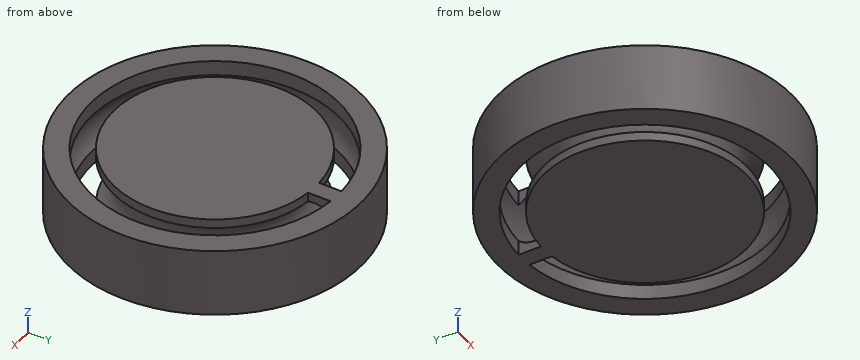
from build123d import *

# Parameters (mm, degrees)
SKETCH_R     = 26
PAD_DEPTH    = 12
POCKET_DEPTH = 12
SKETCH002_R  = 4.5


with BuildPart() as part:
    # Sketch → Pad (new body)
    with BuildSketch(Plane.XY):
        Circle(SKETCH_R)
    extrude(amount=PAD_DEPTH)

    # Sketch001 → Pocket (cut)
    with BuildSketch(Plane.XY):
        with BuildLine():
            ThreePointArc((-1.065198, 21.974197), (-0.435817, -21.995683), (1.934802, 21.914756))
            Line((1.934802, 21.914756), (1.934802, 17.895713))
            ThreePointArc((-1.065198, 17.968454), (-0.436321, -17.994711), (1.934802, 17.895713))
            Line((-1.065198, 21.974197), (-1.065198, 17.968454))
        make_face()
    extrude(amount=POCKET_DEPTH, mode=Mode.SUBTRACT)

    # Sketch002 → Groove (revolve, cut)
    with BuildSketch(Plane.YZ):
        with Locations((19, 6)):
            Circle(SKETCH002_R)
    revolve(axis=Axis((0, 0, 0), (0, 0, 1)), mode=Mode.SUBTRACT)


solid = part.part
Source: CAD feature listing. Evaluate the final solid. Frame: model axes, mm. Give positions to 0.01 mm unless a question says otherwise; leave off trailing zeros. Order: outer loops, then holes, each group sorted by start corner. A loop starts at its lowest first (then second) coordinate and runs counter-clockwise, first axis right, second up. Notation, with made-up numbers: (50.25, 87.25) -> (92.25, 87.25) arc R14 cw to (92.25, 99.25) -> close; hole circle Ø10 at (12.25, 47.5). An arc over 180 degrees is marked (long way). Use a Markdown table: item, result.
1) Section query A-A, the plane z = 3.5. Return the cut outline in (x, y), then the cut area to 3 significant figures.
Answer list:
| item | result |
|---|---|
| outline | circle Ø52 at (0, 0); circle Ø30.52 at (0, 0); hole circle Ø45.48 at (0, 0) |
| area | 1,230 mm² |
2) Contact query for flat-ended pins moving along their axis: P1, Ø3, axis at y = -19, z = 8.5, coming from the -X side; P2, Ø2, axis at x = 13, z = 6, coming from the -Y side; P3, Ø6, axis at x = 1, y = 13, coming from the -Z side; P4, Ø1.3, axis at y = 19, z = 10.5, coming from the +X side. Output: stop coordinate, or through.
Answer list:
| item | result |
|---|---|
| P1 | x = -19.23 |
| P2 | y = -23.07 |
| P3 | z = 0 |
| P4 | x = 18.42 |
3) Section query D-D, the plane z = 7.25. Return the cut outline in (x, y), then the cut area to 3 significant figures.
Answer list:
| item | result |
|---|---|
| outline | circle Ø52 at (0, 0); circle Ø29.35 at (0, 0); hole circle Ø46.65 at (0, 0) |
| area | 1,090 mm² |
4) Section query B-B, the plane y = 3.5. Count the separate pieces of the cut face and the enclosed holes in it, then the cut area to 3 significant figures.
Answer list:
| item | result |
|---|---|
| separate pieces | 3 |
| enclosed holes | 0 |
| area | 460 mm² |
5) Ray query, line 1 along Y through (x, z) = (7, 0.5); line 2 along Y through (x, z) = (8, 11.5); line 3 along X through (y, z) = (-9, 8.5) (3 decimals). Return the intervals inside material, ascending. Write a range as [from, to].
Answer list:
| item | result |
|---|---|
| line 1 | [-25.04, -20.86], [-16.58, 16.58], [20.86, 25.04] |
| line 2 | [-24.74, -20.49], [-16.12, 16.12], [20.49, 24.74] |
| line 3 | [-24.393, -20.885], [-12.321, 12.321], [20.885, 24.393] |
